Could you check a few things on this model? Use its own coordinates, in mm. Give positions to 0.01 mm unless a question says otherwise; leave off trailing zeros. Loops run counter-clockwise (first coordinate to the right, second up) from the corner with the lowest first, then second, coordinate; pieces in that order, holes last. Notation, with made-up numbers: (88.25, 72) - (94.25, 72) arc R19 cw to (94.25, 100) - close; hole circle Ø3 at (64, 89). An arc over 180 degrees is marked (long way). Write each question's results on one line, items separated by ' | '. Start each with the question number.
(1) I need wall thicknesses on line 1 (X direction, y = 2.5, z = 0) (3 decimals); line 2 (Z direction, x = 20, y = 1.8) (3 decimals); line 3 (X direction, y = 2, z = 89). Which ranges of each line are inside material? Lowest first, please.
(2) Suppose I cut it at A-A (x = -71). Please give me the cut outline in (y, z).
(3) For pin 1 (2.5 mm diameter, centred on x = 141, z = 0, fed in from -Y); pin 2 (3 mm diameter, centred on x = 43.5, y = 4.5, fed in from +Z), each with a flat end and sliding along its axis, tell me the tip position at first contact or that it passes through.
(4) If we mould it in two halves opening along Z, with no side actions, what happens to faces 1 (the face through (-2, 5, -1)), 2 (the face through (146.39, 1.01, 101.58)), 3 (the face through (-55.65, 2.54, 91.93))? For each: released by +Z, released by -Z, zero draft, split by the parting line, or undercut.
from build123d import *

# Parameters (mm, degrees)
SKETCH1_W           = 300
SKETCH1_H           = 210
BOSS_EXTRUDE1_DEPTH = 5
FILLET1_R           = 12
SKETCH2_R           = 2.075
CUT_EXTRUDE1_DEPTH  = 6
FILLET2_R           = 3
SKETCH3_R           = 3
SKETCH3_R_2         = 2.56
CUT_EXTRUDE2_DEPTH  = 6


with BuildPart() as part:
    # Sketch1 → Boss-Extrude1 (new body)
    with BuildSketch(Plane(origin=(0, 0, 0), x_dir=(1, 0, 0), z_dir=(0, 1, 0))):
        Rectangle(SKETCH1_W, SKETCH1_H)
    extrude(amount=BOSS_EXTRUDE1_DEPTH)

    # Fillet1
    fillet1_edges = [part.edges().sort_by_distance(p)[0] for p in [
        (150, 2.5, 105),
        (-150, 2.5, 105),
        (-150, 2.5, -105),
        (150, 2.5, -105),
    ]]
    fillet(fillet1_edges, radius=FILLET1_R)

    # Sketch2 → Cut-Extrude1 (cut, through all)
    with BuildSketch(Plane(origin=(0, 5, 0), x_dir=(1, 0, 0), z_dir=(0, 1, 0))):
        with Locations((-141, 70)):
            Circle(SKETCH2_R)
        with Locations((-141, 0)):
            Circle(SKETCH2_R)
        with Locations((-141, -70)):
            Circle(SKETCH2_R)
        with Locations((-20, 70)):
            Circle(SKETCH2_R)
        with Locations((-20, 0)):
            Circle(SKETCH2_R)
        with Locations((-20, -70)):
            Circle(SKETCH2_R)
    cut_extrude1 = extrude(amount=-CUT_EXTRUDE1_DEPTH, mode=Mode.SUBTRACT)

    # Mirror1: Cut-Extrude1 across plane
    add(cut_extrude1.mirror(Plane(origin=(0, 0, 0), x_dir=(0, 0, 1), z_dir=(1, 0, 0))), mode=Mode.SUBTRACT)

    # Fillet2
    fillet2_edges = [part.edges().sort_by_distance(p)[0] for p in [
        (0, 5, -105),
        (150, 5, 0),
        (-150, 5, 0),
        (0, 5, 105),
        (-146.485281374, 5, -101.485281374),
        (-146.485281374, 5, 101.485281374),
        (146.485281374, 5, 101.485281374),
        (146.485281374, 5, -101.485281374),
    ]]
    fillet(fillet2_edges, radius=FILLET2_R)

    # Sketch3 → Cut-Extrude2 (cut, through all)
    with BuildSketch(Plane(origin=(0, 5, 0), x_dir=(1, 0, 0), z_dir=(0, 1, 0))):
        with Locations((-87, -89)):
            Circle(SKETCH3_R)
        with Locations((-71, -89)):
            Circle(SKETCH3_R)
        with Locations((-55, -89)):
            Circle(SKETCH3_R)
        with Locations((-39, -89)):
            Circle(SKETCH3_R_2)
    extrude(amount=-CUT_EXTRUDE2_DEPTH, mode=Mode.SUBTRACT)


solid = part.part
Output values:
1) line 1: -149.958 to -143.075, -138.925 to -22.075, -17.925 to 17.925, 22.075 to 138.925, 143.075 to 149.958 | line 2: -105 to -72.075, -67.925 to -2.075, 2.075 to 67.925, 72.075 to 105 | line 3: -150 to -90, -84 to -74, -68 to -58, -52 to -41.56, -36.44 to 150
2) outline: (0, -105) - (2, -105) arc R3 ccw to (5, -102) - (5, 86) - (0, 86) - close; (0, 92) - (5, 92) - (5, 102) arc R3 ccw to (2, 105) - (0, 105) - close
3) pin 1: through | pin 2: z = 104.83
4) face 1: zero draft | face 2: released by +Z | face 3: undercut
